```python
from build123d import *

# Parameters (mm, degrees)
EXTRUDE_1_DEPTH     = 70
SKETCH_2_R          = 2.3
CUT_EXTRUDE_1_DEPTH = 73.759879054
SKETCH_3_R          = 2.3
CUT_EXTRUDE_2_DEPTH = 73.759879054
CHAMFER_1_SIZE      = 2.05


with BuildPart() as part:
    # Эскиз1 → Бобышка-Вытянуть1 (new body)
    with BuildSketch(Plane(origin=(0, 0, 0), x_dir=(0, 0, -1), z_dir=(1, 0, 0))):
        with BuildLine():
            Line((0, 0), (0, 15))
            Line((0, 15), (1, 15))
            ThreePointArc((1, 15), (1.707106781, 14.707106781), (2, 14))
            Line((2, 14), (2, 3))
            ThreePointArc((2, 3), (2.292893219, 2.292893219), (3, 2))
            Line((3, 2), (14, 2))
            ThreePointArc((14, 2), (14.707106781, 1.707106781), (15, 1))
            Line((15, 1), (15, 0))
            Line((15, 0), (0, 0))
        make_face()
    extrude(amount=EXTRUDE_1_DEPTH)

    # Эскиз2 → Вырез-Вытянуть1 (cut, through all)
    with BuildSketch(Plane(origin=(0, 2, 0), x_dir=(1, 0, 0), z_dir=(0, 1, 0))):
        with Locations(Location((7, 8, 0), (0, 0, 270))):
            Circle(SKETCH_2_R)
        with Locations(Location((63, 8, 0), (0, 0, 270))):
            Circle(SKETCH_2_R)
    extrude(amount=-CUT_EXTRUDE_1_DEPTH, mode=Mode.SUBTRACT)

    # Эскиз3 → Вырез-Вытянуть2 (cut, through all)
    with BuildSketch(Plane(origin=(0, 0, -2), x_dir=(-1, 0, 0), z_dir=(0, 0, -1))):
        with Locations(Location((-16, 8, 0), (0, 0, 90))):
            Circle(SKETCH_3_R)
        with Locations(Location((-54, 8, 0), (0, 0, 90))):
            Circle(SKETCH_3_R)
    extrude(amount=-CUT_EXTRUDE_2_DEPTH, mode=Mode.SUBTRACT)

    # Фаска1
    # the kernel refuses this chamfer: 2.05 mm, written as the material it takes off along each edge
    with BuildSketch(Plane(origin=(63, 0, -8), x_dir=(0, 0, 1), z_dir=(-1, 0, 0))) as chamfer_1_piece_1:
        Polygon((2.3 + CHAMFER_1_SIZE, 0), (2.3, CHAMFER_1_SIZE), (2.3, 0), align=None)
    revolve(axis=Axis((63, 0, -8), (0, 1, 0)), mode=Mode.SUBTRACT)
    with BuildSketch(Plane(origin=(7, 0, -8), x_dir=(0, 0, 1), z_dir=(-1, 0, 0))) as chamfer_1_piece_2:
        Polygon((2.3 + CHAMFER_1_SIZE, 0), (2.3, CHAMFER_1_SIZE), (2.3, 0), align=None)
    revolve(axis=Axis((7, 0, -8), (0, 1, 0)), mode=Mode.SUBTRACT)
    with BuildSketch(Plane(origin=(54, 8, 0), x_dir=(0, 1, 0), z_dir=(-1, 0, 0))) as chamfer_1_piece_3:
        Polygon((2.3 + CHAMFER_1_SIZE, 0), (2.3, CHAMFER_1_SIZE), (2.3, 0), align=None)
    revolve(axis=Axis((54, 8, 0), (0, 0, -1)), mode=Mode.SUBTRACT)
    with BuildSketch(Plane(origin=(16, 8, 0), x_dir=(0, 1, 0), z_dir=(-1, 0, 0))) as chamfer_1_piece_4:
        Polygon((2.3 + CHAMFER_1_SIZE, 0), (2.3, CHAMFER_1_SIZE), (2.3, 0), align=None)
    revolve(axis=Axis((16, 8, 0), (0, 0, -1)), mode=Mode.SUBTRACT)


solid = part.part
```
Work out the finished part from the listing and answer in its coordinate system (mm). A direction names the side the tool comes from. Give positions to 0.01 mm unless a question says otherwise; leave off trailing zeros. Order: outer loops, then holes, each group sorted by start corner. A loop starts at its lowest first (then second) coordinate and runs counter-clockwise, first axis right, second up. Notation, with made-up numbers: (66, 36.25) - (109, 36.25) arc R19 ccw to (109, 51.25) - close; hole circle Ø3 at (36.25, -36). An arc over 180 degrees is marked (long way). One line per item, written item: value. Start each with the question number.
1. Consider line 1 (X direction, y = 6.5, z = -1.5); line 2 (Y direction, x = 53.5, z = -3.5); line 3 (Y direction, x = 51, z = -1). Determine where each line is inside the solid, lowest interval first.
2. Each of these flat-tipped pins is pushed along its axis until it touches: pin 1 Ø3 at (x, y) = (51, 9.5) entering from -Z; pin 2 Ø5.5 at (x, z) = (49.5, -8.5) entering from +Y; pin 3 Ø4 at (y, z) = (5.5, -11) entering from +X. Where does it stop, or does it pass through?
3. Which of the six approach directions +Z, -Z, +X, -X, +Y, -Y give full straight-line access (tool end or side, diameter ignored) to faces 1 (the face through (35, 2, -8)), 2 (the face through (35, 0, -8))?
4. Section D-D, the plane x = 35 is taken. Write down the section's boundary in (y, z).
5. Section A-A, the plane z = -8 is taken. Write down the section's boundary in (x, y).
6. Section C-C, the plane x = 16 is taken. Write down the section's boundary in (y, z).
7. Section B-B, the plane y = 8 is taken. Write down the section's boundary in (x, z), then the cut area to 3 significant figures.
Filled sheet:
1. line 1: 0 to 13.58, 18.42 to 51.58, 56.42 to 70
1. line 2: 0 to 2
1. line 3: 0 to 6.51, 9.49 to 15
2. pin 1: z = -2
2. pin 2: y = 2
2. pin 3: through
3. face 1: -Z, +X, -X, +Y
3. face 2: +Z, -Z, +X, -X, -Y
4. outline: (0, -15) - (1, -15) arc R1 ccw to (2, -14) - (2, -3) arc R1 cw to (3, -2) - (14, -2) arc R1 ccw to (15, -1) - (15, 0) - (0, 0) - close
5. outline: (0, 0) - (2.65, 0) - (4.65, 2) - (0, 2) - close; (9.35, 2) - (11.35, 0) - (58.65, 0) - (60.65, 2) - close; (65.35, 2) - (67.35, 0) - (70, 0) - (70, 2) - close
6. outline: (0, -15) - (1, -15) arc R1 ccw to (2, -14) - (2, -3) arc R1 cw to (3, -2) - (5.65, -2) - (3.65, 0) - (0, 0) - close; (10.35, -2) - (14, -2) arc R1 ccw to (15, -1) - (15, 0) - (12.35, 0) - close
7. outline: (0, -2) - (13.65, -2) - (11.65, 0) - (0, 0) - close; (18.35, -2) - (51.65, -2) - (49.65, 0) - (20.35, 0) - close; (56.35, -2) - (70, -2) - (70, 0) - (58.35, 0) - close
7. area: 113 mm²
